```python
from build123d import *

# Parameters (mm, degrees)
F0_W     = 127
F0_H     = 127
F0_W_2   = 121.92
F0_H_2   = 121.92
F1_DEPTH = 38.1
F1_TAPER = 1.5
F2_W     = 139.7
F2_H     = 139.7
F3_DEPTH = 5.08
F4_R     = 6.35


with BuildPart() as f1:
    # F0 (on Top) → F1 (new body)
    with BuildSketch(Plane.XY):
        Rectangle(F0_W, F0_H)
        Rectangle(F0_W_2, F0_H_2, mode=Mode.SUBTRACT)
    extrude(amount=F1_DEPTH, taper=F1_TAPER)

    # F2 (on Top) → F3 (join)
    with BuildSketch(Plane.XY):
        Rectangle(F2_W, F2_H)
    extrude(amount=-F3_DEPTH)

    # F4
    f4_edges = [f1.edges().sort_by_distance(p)[0] for p in [
        (-69.85, 69.85, -2.54),
        (-69.85, -69.85, -2.54),
        (69.85, -69.85, -2.54),
        (69.85, 69.85, -2.54),
    ]]
    fillet(f4_edges, radius=F4_R)


solid = f1.part
```
The model under review builds one solid part; all positions refer to its coordinate system, in mm. A direction names the side the tool comes from. Round coordinates to 2 decimals unless told otherwise and drop trailing zeros. Put each result on its own line as item: value.
Q1. Machinability: for faces 4 (the flat face through (-6, -67, 0)), 5 (the flat face through (-1, 69.85, -3)), which of the approach directions +Z, -Z, +X, -X, +Y, -Y give a long, thin tool a straight path to every point of the face, cutting with its end or side? Answer none if there is none.
Result set:
face 4: +Z
face 5: +Z, -Z, +X, -X, +Y
Q2. For pin 1 (4 mm diameter, centred on y = 14, z = 26.5, fed in from +X); pin 2 (4 mm diameter, centred on y = 54.5, z = 18, fed in from +X); pin 3 (5 mm diameter, centred on y = -53, z = 30, fed in from +X), all flat-tipped, find the tip position at first contact; note any pin that passes through.
Result set:
pin 1: stops at x = 62.86
pin 2: stops at x = 63.08
pin 3: stops at x = 62.78
Q3. Mouldability with a two-part tool opening along Y and no side actions: class faces 1 (the flat face through (-69.85, -1, -3)), 2 (the flat face through (-1, 1, 0)), 3 (the cylindrical face through (67.94, -68.04, -2.58)) as released by +Y, released by -Y, zero draft, split by the parting line, or undercut.
Result set:
face 1: zero draft
face 2: undercut
face 3: released by -Y
Q4. To check wall thickness, follow L1, parallel to X at y = -1, z = 0.5; L2, parallel to X at y = 19.5, z = 7.5; L3, parallel to Y at x = -44, z = 16. State the ranges of each line that lie inside material, in increasing order.
Result set:
L1: x = -63.49 to -60.97, 60.97 to 63.49
L2: x = -63.3 to -61.16, 61.16 to 63.3
L3: y = -63.08 to -61.38, 61.38 to 63.08
